Job drawing, mm, ordinate dimensions from the low corner. One solid piece. A direction names the side the tool comes from. Give positions to 0.01 mm unless a question says otherwise; leave off trailing zeros. Order: outer loops, then holes, each group sorted by start corner. A loop starts at its lowest first (then second) coordinate and runs counter-clockwise, first axis right, second up. Notation, with made-up numbers: M 28.25,-16.75 L 49.25,-16.75 A21 ccw 49.25,6.25 Z; hole C -27.5,8.5 d2. An arc over 180 degrees is marked long. Put each result on its own line as item: value. Start each with the question number.
1) Cut at C-C (y = 17). Write the cut outline in (x, z).
2) Cut at B-B (z = 54). Write the cut outline in (x, y), and give its area (3 significant figures).
3) Two-plate mould, pull along Y, no slides. Class the marked faces 1, 2 and 3: released by +Y, released by -Y, zero draft, split by the parting line, or undercut.
4) Cut at A-A (x = 26.5). Write the cut outline in (y, z), and give its area (3 significant figures).
5) Drill centre lines: line 1 (Y direction, x = 46.5, z = 7.5); line 2 (Z direction, x = 62.5, y = 22); line 3 (Z direction, x = 30, y = 22.5). Where is each one in solid material? Low to high. Write a range as [from, to].
6) Pin check, flat tips, straight feed: pin 1 (5 mm diameter, centred on y = 22, z = 22, fed in from -X); pin 2 (15 mm diameter, centred on x = 88, y = 19, fed in from +Z); pin 3 (8 mm diameter, centred on y = 9, z = 50, fed in from +X). Stop position of each tip, or through.
7) Cut at D-D (x = 41.5). Write the cut outline in (y, z), and give its area (3 significant figures).
8) Tool access for the marked faces 4, 5 and 6: list every direction of +Z, -Z, +X, -X, +Y, -Y with a clear straight run to the whole face (end or side of a thin tool).
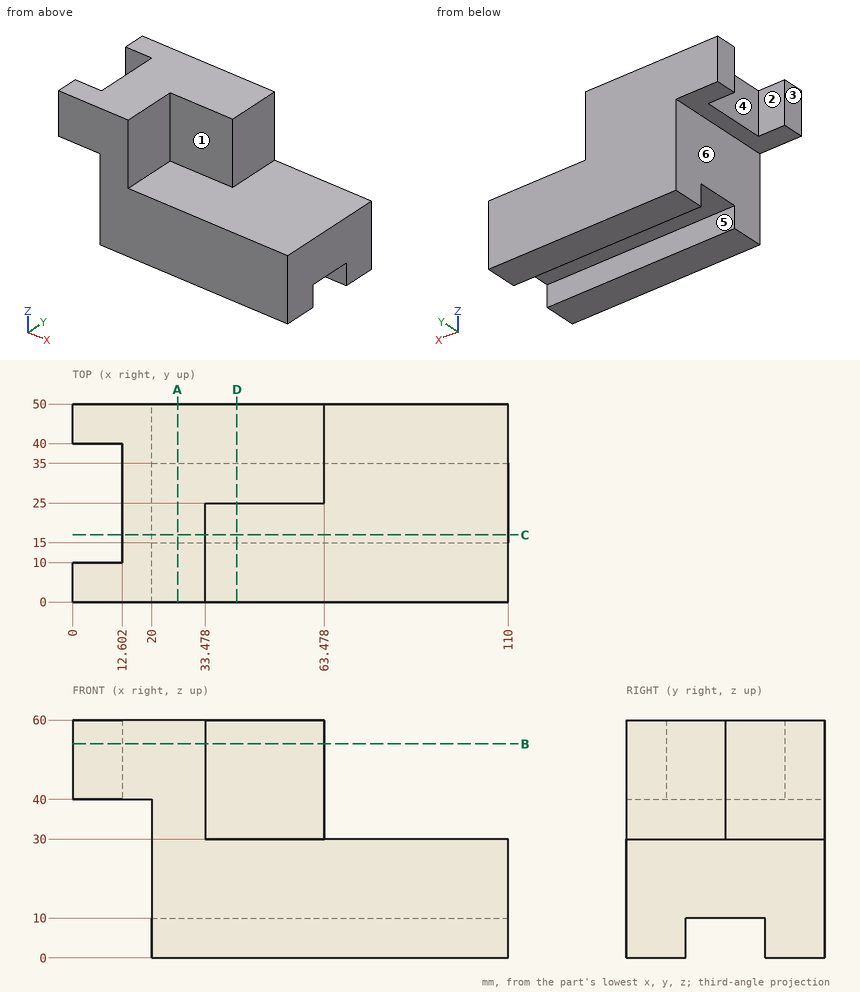
Solution:
1. outline: M 12.6,40 L 20,40 L 20,10 L 110,10 L 110,30 L 33.48,30 L 33.48,60 L 12.6,60 Z
2. outline: M 0,0 L 33.48,0 L 33.48,25 L 63.48,25 L 63.48,50 L 0,50 L 0,40 L 12.6,40 L 12.6,10 L 0,10 Z
2. area: 2,050 mm²
3. face 1: released by -Y
3. face 2: undercut
3. face 3: zero draft
4. outline: M 0,0 L 15,0 L 15,10 L 35,10 L 35,0 L 50,0 L 50,60 L 0,60 Z
4. area: 2,800 mm²
5. line 1: [0, 15], [35, 50]
5. line 2: [10, 30]
5. line 3: [10, 60]
6. pin 1: x = 20
6. pin 2: z = 30
6. pin 3: x = 33.48
7. outline: M 0,0 L 15,0 L 15,10 L 35,10 L 35,0 L 50,0 L 50,60 L 25,60 L 25,30 L 0,30 Z
7. area: 2,050 mm²
8. face 4: +Z, -Z, -X
8. face 5: -Z, +X, -X
8. face 6: -Z, -X, +Y, -Y
